Part model, mm, in its own coordinate system. Give positions to 0.01 mm unless a question says otherwise; leave off trailing zeros. Order: outer loops, then holes, each group sorted by start corner. A loop starts at its lowest first (then second) coordinate and runs counter-clockwise, first axis right, second up. Notation, with made-up numbers: (15.5, 44.5) - (57.5, 44.5) arc R23 cw to (57.5, 63.5) - close; hole circle Ø7 at (-5.75, -17). An arc over 180 degrees is marked (long way). Use one line per item in the form item = value. Start each with the question number.
1. Band-saw the part on D-D, the plane y = 4.2. List the corners of the cut face in (x, z).
2. Pin check, flat tip, straight feed: P1, Ø1, axis at y = 2.5, z = 2, coming from the +X side. Stop position of the tip, or through.
3. Band-saw the part on A-A, the plane x = -0.1. List the corners of the cut face in (y, z) (3 decimals).
4. Pull direction Y, two halves, no side cores. Call faces 1 (the face through (0, 3.18, 2.93)), 2 (the face through (0, 3.57, 2.9)): +Y half, -Y half, draft (parallel to the pull), parting line (faces both ways), or undercut.
5. Band-saw the part on C-C, the plane z = -6.5. List the corners of the cut face in (x, y), plus the area to 3 significant figures.
6. Band-saw the part on B-B, the plane z = 5.75. List the corners of the cut face in (x, y).
7. Drill centre lines: line 1 (Y direction, x = 0.05, z = -7); line 2 (Y direction, x = 0, z = 7.25); line 3 (Y direction, x = 0.15, z = -2.25). Where is each one in solid material? Low to high.
Autodesk Inventor part; units mm, degrees
ref_plane "YZ Plane" through (0, 0, 0) normal (1, 0, 0) x (0, 1, 0)
ref_plane "XZ Plane" through (0, 0, 0) normal (0, 1, 0) x (-1, 0, 0)
ref_plane "XY Plane" through (0, 0, 0) normal (0, 0, 1) x (1, 0, 0)
sketch "Sketch1" plane through (0, 0, 0) normal (0, 1, 0) x (-1, 0, 0)
  line L0 (0.224, 8.675) -> (-0.224, 8.675)
  line L1 (-0.224, 8.675) -> (-0.224, -8.675)
  line L2 (-0.224, -8.675) -> (0.224, -8.675)
  line L3 (0.224, -8.675) -> (0.224, 8.675)
  line L4 (0.224, 8.675) -> (-0.224, -8.675) construction
  line L5 (-0.224, 8.675) -> (0.224, -8.675) construction
  point P0 (0, 0)
  dimension "d0" = 0.448
  dimension "d1" = 17.35
extrude "Plate1" add sketch "Sketch1" along normal blind 0.35
sketch "Sketch2" plane through (0.224, 0.45, 8.775) normal (0, 0, 1) x (1, 0, 0)
  line L0 (-0.448, 0) -> (0, 0)
  line L1 (0, 0) -> (0, 0.3)
  line L2 (0, 0.3) -> (-0.448, 0.3)
  line L3 (-0.448, 0.3) -> (-0.448, 0)
edge flange "Flange1" height 0.75 angle 90 thickness 0.35 bend radius 0.1 thickness toward (0, 0, 1) relief tear relief width 0.35 relief depth 0.175 edges at (0, 0.35, 8.675) wall of the first edge with corners at (-0.224, 0.45, 8.775) (0.224, 0.45, 8.775) (0.224, 0.75, 8.775) (-0.224, 0.75, 8.775)
bend "Bend1"
corner "Corner1"
sketch "Sketch3" plane through (0.224, 0.8427, 8.7125) normal (0, 0.9271839, 0.3746066) x (-1, 0, 0)
  line L0 (0.448, 0) -> (0, 0)
  line L1 (0, 0) -> (0, -12.6465)
  line L2 (0, -12.6465) -> (0.448, -12.6465)
  line L3 (0.448, -12.6465) -> (0.448, 0)
edge flange "Flange2" height 12.95 angle 68 thickness 0.35 bend radius 0.1 thickness toward (0, 0.9271839, 0.3746066) relief tear relief width 0.35 relief depth 0.175 edges at (0, 0.75, 8.775) wall of the first edge with corners at (-0.224, 0.8427, 8.7125) (0.224, 0.8427, 8.7125) (0.224, 5.5802, -3.0131) (-0.224, 5.5802, -3.0131)
bend "Bend2"
corner "Corner2"
equation "\"d2\" = Thickness"
equation "\"d3\" = BendReliefWidth"
equation "\"d4\" = BendReliefDepth"
equation "\"d5\" = MinimumRemnant"
equation "\"d6\" = TransitionRadius"
equation "\"d9\" = BendRadius"
equation "\"d10\" = CornerReliefSize"
equation "\"d11\" = GapSize"
equation "\"d12\" = JacobiRadiusSize"
equation "\"d13\" = BendReliefWidth"
equation "\"d14\" = BendReliefDepth"
equation "\"d15\" = MinimumRemnant"
equation "\"d16\" = TransitionRadius"
equation "\"d19\" = BendRadius"
equation "\"d20\" = CornerReliefSize"
equation "\"d21\" = GapSize"
equation "\"d22\" = JacobiRadiusSize"
equation "\"BendReliefWidth\" = Thickness"
equation "\"BendReliefDepth\" = 0.5 * Thickness"
equation "\"CornerReliefSize\" = 4 * Thickness"
equation "\"MinimumRemnant\" = 2 * Thickness"
equation "\"TransitionRadius\" = BendRadius"
equation "\"JacobiRadiusSize\" = BendRadius"
equation "\"GapSize\" = Thickness"
properties part number "RJ45 Odd Pins" material "Nickel-Copper Alloy 400"
From the geometry:
q1.outline = (-0.22, 0.4) - (0.22, 0.4) - (0.22, 1.34) - (-0.22, 1.34) - close
q2.P1 = through
q3.outline = (0, -8.675) - (0.35, -8.675) - (0.35, 8.675) arc R0.1 cw to (0.45, 8.775) - (0.75, 8.775) arc R0.1 cw to (0.843, 8.712) - (5.58, -3.013) - (5.905, -2.882) - (1.167, 8.844) arc R0.45 ccw to (0.75, 9.125) - (0.45, 9.125) arc R0.45 ccw to (0, 8.675) - close
q4.face_1 = undercut
q4.face_2 = +Y half
q5.outline = (-0.22, 0) - (0.22, 0) - (0.22, 0.35) - (-0.22, 0.35) - close
q5.area = 0.157 mm²
q6.outline = (-0.22, 0) - (0.22, 0) - (0.22, 0.35) - (-0.22, 0.35) - close; (-0.22, 2.04) - (0.22, 2.04) - (0.22, 2.42) - (-0.22, 2.42) - close
q7.line_1 = 0 to 0.35
q7.line_2 = 0 to 0.35, 1.43 to 1.81
q7.line_3 = 0 to 0.35, 5.27 to 5.65
